For this review, take the finished solid that the model builds, in its own axes (mm). A direction names the side the tool comes from. Round coordinates to 2 decimals unless told otherwise and drop trailing zeros. Loops run counter-clockwise (first coordinate to the right, second up) from the corner with the lowest first, then second, coordinate; pieces in that order, holes last.
1. To check wall thickness, follow line 1 along X through (y, z) = (5, 0); line 2 along X through (y, z) = (197, 15); line 3 along X through (y, z) = (10.5, 0). State the ranges of each line that lie inside material, in increasing order.
2. Tool access review of faces 4 (the cylindrical face through (61.198, 12.878, 13.59)), 5 (the cylindrical face through (-17.148, 198.27, -0.477)), 6 (the flat face through (-58, 10, 0)): name each direction out of +Z, -Z, +X, -X, +Y, -Y from which nothing blocks a thin tool from reaching the whole face with its end or side.
3. Clearance check with flat-ended pins moving along their axes: pin 1 Ø8 at (y, z) = (104, 36) entering from -X; pin 2 Ø2 at (y, z) = (105.5, -24.5) entering from +X; pin 3 Ø4 at (x, y) = (-13, 135.5) entering from +Z. State where each tip first meets the part, or that it passes through.
4. Consider section D-D on y = 150. State the section outline as (x, z) points, then the cut area to 3 significant figures.
5. Draft analysis for pull direction Z (two halves, no side actions). For faces 1 (the flat face through (-51.4, 0, -0.3)), 2 (the cylindrical face through (55.835, 4.93, 0.477)), 3 (the conical face through (40.738, 115.545, 9.046)), state which applies: released by +Z, released by -Z, zero draft, split by the parting line, or undercut.
6. Consider section C-C on y = 17. State the section outline as (x, z) points.
from build123d import *

# Parameters (mm, degrees)
SKETCH3_R          = 2.2
CUT_EXTRUDE1_DEPTH = 10
SKETCH4_R          = 2.2
CUT_EXTRUDE2_DEPTH = 10


with BuildPart() as part:
    # Sketch2 → Revolve1 (revolve)
    with BuildSketch(Plane.XY, mode=Mode.PRIVATE) as revolve1_sk:
        Polygon((50.8635, 0), (62.6885, 0), (62.6885, 25.4), (21.35, 203.2), (6.35, 203.2), (47.6885, 25.4), (47.6885, 4.064), (50.8635, 4.064), align=None)
    revolve(revolve1_sk.sketch.rotate(Axis((0, 0, 0), (0, 1, 0)), 90), axis=Axis((0, 0, 0), (0, 1, 0)))

    # Sketch3 → Cut-Extrude1 (cut)
    with BuildSketch(Plane.XZ):
        with Locations(Location((-57.9825, 0, 0), (0, 0, 270))):
            Circle(SKETCH3_R)
        with Locations(Location((0, 57.9825, 0), (0, 0, 270))):
            Circle(SKETCH3_R)
        with Locations(Location((57.9825, 0, 0), (0, 0, 270))):
            Circle(SKETCH3_R)
        with Locations(Location((0, -57.9825, 0), (0, 0, 270))):
            Circle(SKETCH3_R)
    extrude(amount=-CUT_EXTRUDE1_DEPTH, mode=Mode.SUBTRACT)

    # Sketch4 → Cut-Extrude2 (cut)
    with BuildSketch(Plane(origin=(0, 203.2, 0), x_dir=(1, 0, 0), z_dir=(0, 1, 0))):
        with Locations(Location((-15, 0, 0), (0, 0, 270))):
            Circle(SKETCH4_R)
        with Locations(Location((0, 15, 0), (0, 0, 270))):
            Circle(SKETCH4_R)
        with Locations(Location((15, 0, 0), (0, 0, 270))):
            Circle(SKETCH4_R)
        with Locations(Location((0, -15, 0), (0, 0, 270))):
            Circle(SKETCH4_R)
    extrude(amount=-CUT_EXTRUDE2_DEPTH, mode=Mode.SUBTRACT)


solid = part.part
Resolved:
1. line 1: x = -62.69 to -60.18, -55.78 to -47.69, 47.69 to 55.78, 60.18 to 62.69
1. line 2: x = -17.16 to -2.2, 2.2 to 17.16
1. line 3: x = -62.69 to -47.69, 47.69 to 62.69
2. face 4: +Y, -Y
2. face 5: +Y
2. face 6: -Y
3. pin 1: stops at x = -31.01
3. pin 2: stops at x = 37.33
3. pin 3: stops at z = 35.59
4. outline: circle Ø67.44 at (0, 0); hole circle Ø37.44 at (0, 0)
4. area: 2,470 mm2
5. face 1: zero draft
5. face 2: undercut
5. face 3: split by the parting line
6. outline: circle Ø125.38 at (0, 0); hole circle Ø95.38 at (0, 0)
